from build123d import *

# Parameters (mm, degrees)
F1_DEPTH = 2.54
F3_DEPTH = 25.4
F5_DEPTH = 25.4


with BuildPart() as f1:
    # F0 (on Top) → F1 (new body)
    with BuildSketch(Plane.XY):
        Polygon((31.749999, -122.967221), (122.367737, -33.987305), (90.617738, 88.979917), (-31.749999, 122.967221), (-122.367737, 33.987305), (-90.617738, -88.979917), align=None)
    extrude(amount=F1_DEPTH)

    # F2 (on face) → F3 (cut)
    with BuildSketch(Plane.XY.offset(2.54)):
        Polygon((-90.617738, -88.979917), (90.617738, 88.979917), (-31.749999, 122.967221), (-122.367737, 33.987305), align=None)
    extrude(amount=-F3_DEPTH, mode=Mode.SUBTRACT)

    # F4 (on face) → F5 (cut)
    with BuildSketch(Plane.XY.offset(2.54)):
        with BuildLine():
            ThreePointArc((-63.432417, -62.285942), (33.645714, -82.287155), (88.9, 0))
            ThreePointArc((88.9, 0), (82.287155, 33.645714), (63.432417, 62.285942))
            Line((63.432417, 62.285942), (-63.432417, -62.285942))
        make_face()
    extrude(amount=-F5_DEPTH, mode=Mode.SUBTRACT)


solid = f1.part
The listing builds one solid part. Answer for the finished solid, in the listing's coordinates (mm). Coordinates: 2 decimals unless noted, no trailing zeros. Loops run counter-clockwise (first coordinate to the right, second up) from the corner with the lowest first, then second, coordinate; pieces in that order, holes last.
1) Find the intervals of material crossed by L1, parallel to X at y = -68.5, z = 1.25; L2, parallel to X at y = 35, z = 0.65; L3, parallel to Y at x = -45.5, z = 1.6, in increasing order.
2) Find section A-A on z = 1.55. Write down the section's boundary in (x, y).
3) Find section C-C on y = 49.5. Write down the section's boundary in (x, z), then the cut area to 3 significant figures.
4) Find section B-B on x = 45.5. Write down the section's boundary in (y, z).
5) Flat-ended cylindrical pins translate along their axes: pin 1 Ø1 at (y, z) = (16, 2) entering from +X; pin 2 Ø1 at (x, z) = (-46.5, 1.5) entering from -Y. Find the tip coordinate at first contact, or state that the pin passes through.
Values:
1. L1: x = -69.76 to -56.67, 56.67 to 87.22
1. L2: x = 81.72 to 104.56
1. L3: y = -101.51 to -76.37
2. outline: (-90.62, -88.98) - (31.75, -122.97) - (122.37, -33.99) - (90.62, 88.98) - (63.43, 62.29) arc R88.9 cw to (88.9, 0) arc R88.9 cw to (-63.43, -62.29) - close
3. outline: (73.84, 0) - (100.81, 0) - (100.81, 2.54) - (73.84, 2.54) - close
3. area: 68.5 mm2
4. outline: (-109.47, 0) - (-76.37, 0) - (-76.37, 2.54) - (-109.47, 2.54) - close
5. pin 1: stops at x = 109.59
5. pin 2: stops at y = -101.37
